Design review of the part built by this model. Coordinates are the model's own, in mm. Face numbers are marked on the shaded views. A direction names the side the tool comes from. Give positions to 0.01 mm unless a question says otherwise; leave off trailing zeros. Loops run counter-clockwise (first coordinate to the right, second up) from the corner with the lowest first, then second, coordinate; pieces in that order, holes last. Notation, with made-up numbers: (59, 85.5) -> (82, 85.5) arc R33 ccw to (82, 116.5) -> close; hole circle Ø9 at (77.25, 50.5). An arc over 180 degrees is marked (long way). Answer as CSV lines item,"result".
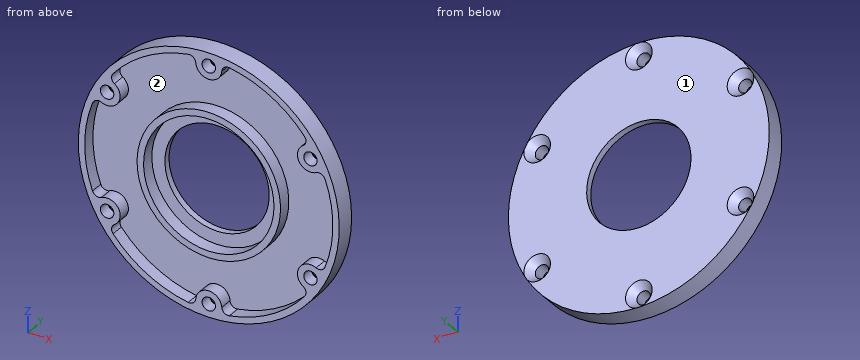
from build123d import *

# Parameters (mm, degrees)
SKETCH1_R                                         = 31.75
BOSS_EXTRUDE1_DEPTH                               = 4.7625
CSK_FOR_4_FLAT_HEAD_SOCKET_CAP_SCREW1_D           = 3.2639
CSK_FOR_4_FLAT_HEAD_SOCKET_CAP_SCREW1_CSINK_D     = 6.477
CSK_FOR_4_FLAT_HEAD_SOCKET_CAP_SCREW1_CSINK_ANGLE = 82
SKETCH6_R                                         = 15.875
CUT_EXTRUDE1_DEPTH                                = 3.175
SKETCH7_R                                         = 12.7
CUT_EXTRUDE2_DEPTH                                = 3.175
SKETCH8_R                                         = 17.4625
CUT_EXTRUDE3_DEPTH                                = 3.175


with BuildPart() as part:
    # Sketch1 → Boss-Extrude1 (new body)
    with BuildSketch(Plane(origin=(0, 0, 0), x_dir=(1, 0, 0), z_dir=(0, 1, 0))):
        with Locations(Location((0, 0, 0), (0, 0, 90))):
            Circle(SKETCH1_R)
    extrude(amount=BOSS_EXTRUDE1_DEPTH)

    # CSK for #4 Flat Head Socket Cap Screw1 (through all)
    with Locations(Plane(origin=(0, 4.7625, 0), x_dir=(-1, 0, 0), z_dir=(0, 1, 0))):
        with Locations((0, 28.575), (24.746675913, 14.2875), (24.746675913, -14.2875), (0, -28.575), (-24.746675913, -14.2875), (-24.746675913, 14.2875)):
            CounterSinkHole(CSK_FOR_4_FLAT_HEAD_SOCKET_CAP_SCREW1_D / 2, CSK_FOR_4_FLAT_HEAD_SOCKET_CAP_SCREW1_CSINK_D / 2, counter_sink_angle=CSK_FOR_4_FLAT_HEAD_SOCKET_CAP_SCREW1_CSINK_ANGLE)

    # Sketch6 → Cut-Extrude1 (cut)
    with BuildSketch(Plane.XZ):
        with Locations(Location((0, 0, 0), (0, 0, 270))):
            Circle(SKETCH6_R)
    extrude(amount=-CUT_EXTRUDE1_DEPTH, mode=Mode.SUBTRACT)

    # Sketch7 → Cut-Extrude2 (cut)
    with BuildSketch(Plane.XZ.offset(-3.175)):
        with Locations(Location((0, 0, 0), (0, 0, 270))):
            Circle(SKETCH7_R)
    extrude(amount=-CUT_EXTRUDE2_DEPTH, mode=Mode.SUBTRACT)

    # Sketch8 → Cut-Extrude3 (cut)
    with BuildSketch(Plane.XZ):
        with BuildLine():
            ThreePointArc((26.134754006, 11.432002809), (27.408069158, 11.477856343), (28.298548725, 10.5665495))
            ThreePointArc((28.298548725, 10.5665495), (30.20695, 0), (28.298548725, -10.5665495))
            ThreePointArc((28.298548725, -10.5665495), (27.408069158, -11.477856343), (26.134754006, -11.432002809))
            ThreePointArc((26.134754006, -11.432002809), (21.997045256, -12.7), (22.967781852, -16.917359487))
            ThreePointArc((22.967781852, -16.917359487), (23.644149753, -17.997155988), (23.30017466, -19.223987337))
            ThreePointArc((23.30017466, -19.223987337), (15.103475, -26.159986071), (4.998374065, -29.790536836))
            ThreePointArc((4.998374065, -29.790536836), (3.763919405, -29.475012331), (3.166972154, -28.349362296))
            ThreePointArc((3.166972154, -28.349362296), (0, -25.4), (-3.166972154, -28.349362296))
            ThreePointArc((-3.166972154, -28.349362296), (-3.763919405, -29.475012331), (-4.998374065, -29.790536836))
            ThreePointArc((-4.998374065, -29.790536836), (-15.103475, -26.159986071), (-23.30017466, -19.223987337))
            ThreePointArc((-23.30017466, -19.223987337), (-23.644149753, -17.997155988), (-22.967781852, -16.917359487))
            ThreePointArc((-22.967781852, -16.917359487), (-21.997045256, -12.7), (-26.134754006, -11.432002809))
            ThreePointArc((-26.134754006, -11.432002809), (-27.408069158, -11.477856343), (-28.298548725, -10.5665495))
            ThreePointArc((-28.298548725, -10.5665495), (-30.20695, 0), (-28.298548725, 10.5665495))
            ThreePointArc((-28.298548725, 10.5665495), (-27.408069158, 11.477856343), (-26.134754006, 11.432002809))
            ThreePointArc((-26.134754006, 11.432002809), (-21.997045256, 12.7), (-22.967781852, 16.917359487))
            ThreePointArc((-22.967781852, 16.917359487), (-23.644149753, 17.997155988), (-23.30017466, 19.223987337))
            ThreePointArc((-23.30017466, 19.223987337), (-15.103475, 26.159986071), (-4.998374065, 29.790536836))
            ThreePointArc((-4.998374065, 29.790536836), (-3.763919405, 29.475012331), (-3.166972154, 28.349362296))
            ThreePointArc((-3.166972154, 28.349362296), (0, 25.4), (3.166972154, 28.349362296))
            ThreePointArc((3.166972154, 28.349362296), (3.763919405, 29.475012331), (4.998374065, 29.790536836))
            ThreePointArc((4.998374065, 29.790536836), (15.103475, 26.159986071), (23.30017466, 19.223987337))
            ThreePointArc((23.30017466, 19.223987337), (23.644149753, 17.997155988), (22.967781852, 16.917359487))
            ThreePointArc((22.967781852, 16.917359487), (21.997045256, 12.7), (26.134754006, 11.432002809))
        make_face()
        with Locations(Location((0, 0, 0), (0, 0, 270))):
            Circle(SKETCH8_R, mode=Mode.SUBTRACT)
    extrude(amount=-CUT_EXTRUDE3_DEPTH, mode=Mode.SUBTRACT)


solid = part.part
Q1. We need section C-C, the plane z = -23. State the section outline as (x, y) points (1 decimal).
Filled sheet:
outline,"(-21.9, 0) -> (-19.6, 0) -> (-19.6, 3.2) -> (19.6, 3.2) -> (19.6, 0) -> (21.9, 0) -> (21.9, 4.8) -> (-21.9, 4.8) -> close"
Q2. For the marked faces 1 and 2, list the 3-axis set-ups (+Z, -Z, +X, -X, +Y, -Y) from which the entire face can be reached by the end or side of a thin tool; tool diameter is ignored.
Filled sheet:
face 1,"+Z, -Z, +X, -X, +Y"
face 2,"-Y"
Q3. Clearance check with flat-ended pins moving along their axes: pin 1 Ø5 at (x, z) = (0, 28.575) entering from -Y; pin 2 Ø19 at (x, z) = (0, 0) entering from -Y; pin 3 Ø4 at (x, z) = (0, -28.575) entering from +Y; pin 4 Ø2 at (y, z) = (2.5, -24) entering from -X. State where each tip first meets the part, or that it passes through.
Filled sheet:
pin 1,"stops at y = 0"
pin 2,"passes through"
pin 3,"stops at y = 3.34"
pin 4,"stops at x = -21.89"
Q4. To check wall thickness, follow probe 1 along X at (y, z) = (4.1, 0); probe 2 along Z at (x, y) = (12, 1); probe 3 along X at (y, z) = (2.95, 0.5). State the ranges of each line that lie inside material, in increasing order. Write a range as from..to.
Filled sheet:
probe 1,"x = -31.75..-12.7, 12.7..31.75"
probe 2,"z = -29.39..-27.72, -12.69..-10.39, 10.39..12.69, 27.72..29.39"
probe 3,"x = -31.75..-30.2, -17.46..-15.87, 15.87..17.46, 30.2..31.75"
Q5. We need section B-B, the plane y = 1.3. State how many separate pieces and enclosed holes the cut face has, and give its area (3 significant figures).
Filled sheet:
separate pieces,"2"
enclosed holes,"8"
area,"580 mm^2"
